The model under review builds one solid part; all positions refer to its coordinate system, in mm. Face numbers are marked on the shaded views. A direction names the side the tool comes from. Give positions to 0.01 mm unless a question says otherwise; leave off trailing zeros. Loops run counter-clockwise (first coordinate to the right, second up) from the corner with the lowest first, then second, coordinate; pieces in that order, holes last. Notation, with made-up numbers: M 81,-24 L 93,-24 A20 ccw 93,-18 Z; hole C 53.5,54.5 d9. An arc over 180 degrees is marked long. Write item = value, one per line. Start each with the question number.
1. For the marked faces 1 and 2, list the 3-axis set-ups (+Z, -Z, +X, -X, +Y, -Y) from which the entire face can be reached by the end or side of a thin tool; tool diameter is ignored.
2. We need section C-C on x = -33.5. Give the boundary of the cut face in (y, z).
3. We need section B-B on y = 37. Give the boundary of the cut face in (x, z), then the cut area to 3 significant figures.
4. Draft analysis for pull direction Z (two halves, no side actions). For the marked faces 3 and 4, state which applies: pulls with the +Z half, pulls with the -Z half, needs draft (parallel to the pull), parting line crosses it, or undercut.
5. For pin 1 (3 mm diameter, centred on x = -23, y = 38.21, fed in from +Z); pin 2 (6.5 mm diameter, centred on x = -76, z = -9, fed in from +Y); pin 3 (3 mm diameter, centred on x = -43.2, y = 29.31, fed in from +Z); pin 4 (4 mm diameter, centred on x = -38, z = -6.5, fed in from -Y), all flat-tipped, find the tip position at first contact; note any pin that passes through.
6. We need section D-D on x = -59.55. Give the boundary of the cut face in (y, z), then the cut area to 3 significant figures.
7. Wall thickness on line 1 along Y through (x, z) = (-39.35, -13.1); line 2 along Y through (x, z) = (-48.05, -12.95); line 3 along Y through (x, z) = (-59.55, -13.2): over which ranges is each line inside the solid? List them lowest first. Write a range as from..to.
8. We need section A-A on z = -9. Count the separate pieces of the cut face and the enclosed holes in it, then the cut area to 3 significant figures.
from build123d import *

# Parameters (mm, degrees)
SKETCH1_R             = 1.5875
BOSS_EXTRUDE1_DEPTH   = 1.5875
SKETCH1_W             = 12.7
SKETCH1_H             = 12.7
BOSS_EXTRUDE1_2_DEPTH = 1.5875
SKETCH2_W             = 69.85
SKETCH2_H             = 53
BOSS_EXTRUDE2_DEPTH   = 1.5875
BOSS_EXTRUDE3_DEPTH   = 1.5875
SKETCH6_W             = 1.5875
SKETCH6_H             = 53
BOSS_EXTRUDE4_DEPTH   = 12.7
SKETCH7_W             = 12.7
SKETCH7_H             = 12.7
CUT_EXTRUDE1_DEPTH    = 12.7
SKETCH10_W            = 13.49375
SKETCH10_H            = 0.79375
CUT_EXTRUDE3_DEPTH    = 100.134429722
SKETCH13_R            = 1.25
SKETCH13_R_2          = 3
SKETCH13_R_3          = 2.000000064
CUT_EXTRUDE4_DEPTH    = 12.7
FILLET1_R             = 6.35
FILLET2_R             = 6.35
SKETCH14_W            = 12.7
SKETCH14_H            = 12.7
SKETCH14_R            = 1.5875
BOSS_EXTRUDE5_DEPTH   = 0.79375
FILLET3_R             = 6.35
SKETCH15_R            = 1.6
CUT_EXTRUDE7_DEPTH    = 0.79375


with BuildPart() as part:
    # Sketch1 → Boss-Extrude1 (new body)
    with BuildSketch(Plane(origin=(0, 0, 0), x_dir=(1, 0, 0), z_dir=(0, 1, 0))):
        Polygon((-12.7, 0), (0, 0), (0, 12.7), (-12.7, 12.7), (-12.7, 6.35), align=None)
        with Locations(Location((-6.35, 6.35, 0), (0, 0, 270))):
            Circle(SKETCH1_R, mode=Mode.SUBTRACT)
    extrude(amount=BOSS_EXTRUDE1_DEPTH)



with BuildPart() as body_2:
    # Sketch1 → Boss-Extrude1 2 (new body)
    with BuildSketch(Plane(origin=(0, 0, 0), x_dir=(1, 0, 0), z_dir=(0, 1, 0))):
        with Locations((-63.5, 6.35)):
            Rectangle(SKETCH1_W, SKETCH1_H)
        with Locations(Location((-63.5, 6.35, 0), (0, 0, 270))):
            Circle(SKETCH1_R, mode=Mode.SUBTRACT)
    extrude(amount=BOSS_EXTRUDE1_2_DEPTH)


with BuildPart() as part_1:
    add(part.part)

    add(body_2.part)  # Boss-Extrude2 merges body 2
    # Sketch2 → Boss-Extrude2 (add)
    with BuildSketch(Plane(origin=(0, 0, -12.7), x_dir=(-1, 0, 0), z_dir=(0, 0, -1))):
        with Locations((34.925, 26.5)):
            Rectangle(SKETCH2_W, SKETCH2_H)
    extrude(amount=BOSS_EXTRUDE2_DEPTH)

    # Sketch5 → Boss-Extrude3 (add)
    with BuildSketch(Plane(origin=(0, 1.5875, 0), x_dir=(1, 0, 0), z_dir=(0, 1, 0))):
        with BuildLine():
            Line((-69.85, 0), (-69.85, 6.35))
            Line((-69.85, 6.35), (-74.6125, 6.35))
            ThreePointArc((-74.6125, 6.35), (-76.2, 4.7625), (-77.7875, 6.35))
            Line((-77.7875, 6.35), (-82.55, 6.35))
            Line((-82.55, 6.35), (-82.55, 0))
            Line((-82.55, 0), (-69.85, 0))
        make_face()
        with BuildLine():
            ThreePointArc((-77.7875, 6.35), (-77.322532015, 7.472532015), (-76.2, 7.9375))
            Line((-76.2, 7.9375), (-76.2, 12.7))
            Line((-76.2, 12.7), (-82.55, 12.7))
            Line((-82.55, 12.7), (-82.55, 6.35))
            Line((-82.55, 6.35), (-77.7875, 6.35))
        make_face()
        with BuildLine():
            Line((-74.6125, 6.35), (-69.85, 6.35))
            Line((-69.85, 6.35), (-69.85, 12.7))
            Line((-69.85, 12.7), (-76.2, 12.7))
            Line((-76.2, 12.7), (-76.2, 7.9375))
            ThreePointArc((-76.2, 7.9375), (-75.077467985, 7.472532015), (-74.6125, 6.35))
        make_face()
    extrude(amount=-BOSS_EXTRUDE3_DEPTH)

    # Sketch6 → Boss-Extrude4 (add)
    with BuildSketch(Plane.ZY.offset(69.85)):
        with Locations((-13.49375, 26.5)):
            Rectangle(SKETCH6_W, SKETCH6_H)
    extrude(amount=BOSS_EXTRUDE4_DEPTH)

    # Sketch7 → Cut-Extrude1 (cut)
    with BuildSketch(Plane(origin=(0, 1.5875, 0), x_dir=(1, 0, 0), z_dir=(0, 1, 0))):
        with Locations((-63.5, 6.35)):
            Rectangle(SKETCH7_W, SKETCH7_H)
    extrude(amount=-CUT_EXTRUDE1_DEPTH, mode=Mode.SUBTRACT)

    # Sketch10 → Cut-Extrude3 (cut, through all)
    with BuildSketch(Plane(origin=(0, 0, 0), x_dir=(0, 0, -1), z_dir=(1, 0, 0))):
        with Locations((6.746875, 0.396875)):
            Rectangle(SKETCH10_W, SKETCH10_H)
        Polygon((13.49375, 0.79375), (13.49375, 0), (14.2875, 0), (14.2875, 53), (13.49375, 53), align=None)
    extrude(amount=-CUT_EXTRUDE3_DEPTH, mode=Mode.SUBTRACT)

    # Sketch13 → Cut-Extrude4 (cut)
    with BuildSketch(Plane(origin=(0, 0, -13.49375), x_dir=(-1, 0, 0), z_dir=(0, 0, -1))):
        with Locations((43.2, 24.48749994)):
            Circle(SKETCH13_R)
        with Locations((43.2, 6.68749994)):
            Circle(SKETCH13_R)
        with Locations((34.5, 15.58749994)):
            Circle(SKETCH13_R_2)
        with Locations((23, 15.58749994)):
            Circle(SKETCH13_R_3)
        with Locations((39.35, 6.68749994)):
            Circle(SKETCH13_R)
        with Locations((39.35, 24.48749994)):
            Circle(SKETCH13_R)
        with Locations((48.05, 15.58749994)):
            Circle(SKETCH13_R_2)
        with Locations((59.55, 15.58749994)):
            Circle(SKETCH13_R_3)
        with Locations((59.55, 38.20625006)):
            Circle(SKETCH13_R_3)
        with Locations((48.05, 38.20625006)):
            Circle(SKETCH13_R_2)
        with Locations((39.35, 29.30625006)):
            Circle(SKETCH13_R)
        with Locations(Location((39.35, 47.10625006, 0), (0, 0, 180))):
            Circle(SKETCH13_R)
        with Locations((23, 38.20625006)):
            Circle(SKETCH13_R_3)
        with Locations((34.5, 38.20625006)):
            Circle(SKETCH13_R_2)
        with Locations((43.2, 47.10625006)):
            Circle(SKETCH13_R)
        with Locations((43.2, 29.30625006)):
            Circle(SKETCH13_R)
    extrude(amount=-CUT_EXTRUDE4_DEPTH, mode=Mode.SUBTRACT)

    # Fillet1
    fillet1_edges = [part_1.edges().sort_by_distance(p)[0] for p in [
        (-12.7, 1.190625, 0),
        (0, 1.190625, 0),
    ]]
    fillet(fillet1_edges, radius=FILLET1_R - 0.0001)  # a hair under: the kernel refuses the full size

    # Fillet2
    fillet2_edges = [part_1.edges().sort_by_distance(p)[0] for p in [
        (-82.55, 1.190625, 0),
        (-69.85, 1.190625, 0),
    ]]
    fillet(fillet2_edges, radius=FILLET2_R - 0.0001)  # a hair under: the kernel refuses the full size

    # Sketch14 → Boss-Extrude5 (add)
    with BuildSketch(Plane(origin=(0, 53, 0), x_dir=(1, 0, 0), z_dir=(0, 1, 0))):
        with Locations((-41.275, 6.35)):
            Rectangle(SKETCH14_W, SKETCH14_H)
        with Locations(Location((-41.275, 6.35, 0), (0, 0, 270))):
            Circle(SKETCH14_R, mode=Mode.SUBTRACT)
    extrude(amount=-BOSS_EXTRUDE5_DEPTH)

    # Fillet3
    fillet3_edges = [part_1.edges().sort_by_distance(p)[0] for p in [
        (-47.625, 52.603125, 0),
        (-34.925, 52.603125, 0),
    ]]
    fillet(fillet3_edges, radius=FILLET3_R - 0.0001)  # a hair under: the kernel refuses the full size

    # Sketch15 → Cut-Extrude7 (cut)
    with BuildSketch(Plane(origin=(0, 0, -13.49375), x_dir=(-1, 0, 0), z_dir=(0, 0, -1))):
        with Locations((22.775, 43.862031033)):
            Circle(SKETCH15_R)
        with Locations((22.775, 9.931718967)):
            Circle(SKETCH15_R)
        with Locations((59.775, 9.931718967)):
            Circle(SKETCH15_R)
        with Locations((59.775, 43.862031033)):
            Circle(SKETCH15_R)
    extrude(amount=-CUT_EXTRUDE7_DEPTH, mode=Mode.SUBTRACT)


solid = part_1.part
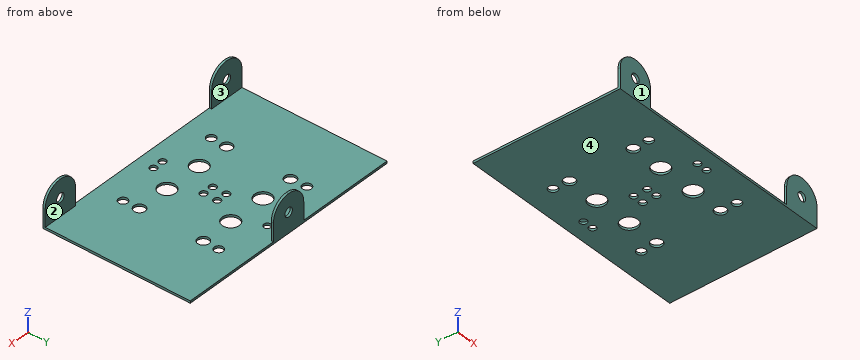
Final values:
q1.face_1 = +Z, -Z, +X, -X, -Y
q1.face_2 = +Z, +X, -X, +Y
q2.outline = M 0.79,-13.49 L 12.76,-13.49 L 12.76,-12.7 L 0.79,-12.7 Z; M 18.42,-13.49 L 35.38,-13.49 L 35.38,-12.7 L 18.42,-12.7 Z; M 41.03,-13.49 L 53,-13.49 L 53,-12.7 L 41.03,-12.7 Z
q3.outline = M -82.55,-13.49 L -61.15,-13.49 L -61.15,-12.7 L -82.55,-12.7 Z; M -57.95,-13.49 L -50.8,-13.49 L -50.8,-12.7 L -57.95,-12.7 Z; M -45.3,-13.49 L -37.25,-13.49 L -37.25,-12.7 L -45.3,-12.7 Z; M -31.75,-13.49 L -24.6,-13.49 L -24.6,-12.7 L -31.75,-12.7 Z; M -21.4,-13.49 L 0,-13.49 L 0,-12.7 L -21.4,-12.7 Z
q3.area = 51.7 mm²
q4.face_3 = needs draft
q4.face_4 = pulls with the -Z half
q5.pin_1 = through
q5.pin_2 = 1.59
q5.pin_3 = -12.7
q5.pin_4 = 52.21
q6.outline = M 0.79,-13.49 L 8.35,-13.49 L 8.35,-12.7 L 0.79,-12.7 Z; M 11.52,-13.49 L 13.59,-13.49 L 13.59,-12.7 L 11.52,-12.7 Z; M 17.59,-13.49 L 36.21,-13.49 L 36.21,-12.7 L 17.59,-12.7 Z; M 40.21,-13.49 L 42.28,-13.49 L 42.28,-12.7 L 40.21,-12.7 Z; M 45.45,-13.49 L 53,-13.49 L 53,-12.7 L 45.45,-12.7 Z
q6.area = 30.1 mm²
q7.line_1 = 0.79..5.44, 7.94..23.24, 25.74..28.06, 30.56..45.86, 48.36..53
q7.line_2 = 0.79..12.59, 18.59..35.21, 41.21..53
q7.line_3 = 0.79..8.35, 11.52..13.59, 17.59..36.21, 40.21..42.28, 45.45..53
q8.separate_pieces = 3
q8.enclosed_holes = 0
q8.area = 30.2 mm²
